The listing builds one solid part. Answer for the finished solid, in the listing's coordinates (mm). A direction names the side the tool comes from. Round coordinates to 2 decimals unless told otherwise and drop trailing zeros. Write each loop counter-clockwise with the first axis right and the second up, starting at its lowest first coordinate (ties: lowest second). Pieces come first, ordered by that corner, then holes. Notation, with made-up numbers: (39.5, 21) - (86.5, 21) arc R24 cw to (86.5, 43) - close; hole circle Ø7 at (-40, 82). An arc over 180 degrees is marked (long way). Return JSON: item names as keys, results as strings. Group by question number.
(1) Section D-D, the plane x = 7.75 is taken. Write down the section's boundary in (y, z), then the cut area to 3 significant figures.
(2) Section C-C, the plane z = 71 is taken. Write down the section's boundary in (x, y), then the cut area to 3 significant figures.
(3) Find the intervals of material crossed by line 1 along Z through (x, y) = (15, 1.4); line 2 along Y through (x, z) = (14.25, 40), in increasing order. Write a range as [from, to].
(4) Which of the six approach directions +Z, -Z, +X, -X, +Y, -Y give full straight-line access (tool end or side, diameter ignored) to faces 1 (the flat face through (16, 2.5, 93)), 2 (the cylindrical face through (1.27, 12.05, 17.7))?
(5) Determine the mould class of faces 3 (the cylindrical face through (15.867, 1.268, 171.895)), 4 (the cylindrical face through (18.996, 1.268, 12.676)), 5 (the flat face through (15, 0, 93)), 6 (the flat face through (2.5, 16, 93)) for opening direction X: +X half, -X half, draft (parallel to the pull), parting line (faces both ways), or undercut.
(6) Section B-B, the plane x = 15 is taken. Write down the section's boundary in (y, z), then the cut area to 3 significant figures.
(7) Each of these flat-tipped pins is pushed along its axis until it touches: pin 1 (13 mm diameter, centred on x = 15, z = 12.5, fed in from +Y); pin 2 (9 mm diameter, centred on y = 15, z = 15, fed in from +X); pin 3 (7 mm diameter, centred on x = 15, z = 175.8, fed in from -Y). Where does it stop, or does it pass through?
(8) Section A-A, the plane y = 15 is taken. Write down the section's boundary in (x, z).
```python
from build123d import *

# Parameters (mm, degrees)
BOSS_EXTRUDE1_DEPTH = 188.3
SKETCH2_R           = 4
CUT_EXTRUDE1_DEPTH  = 193.647709563
SKETCH3_R           = 4
CUT_EXTRUDE2_DEPTH  = 193.647709563


with BuildPart() as part:
    # Sketch1 → Boss-Extrude1 (new body)
    with BuildSketch(Plane.XY):
        Polygon((0, 0), (0, 30), (2.5, 30), (2.5, 2.5), (30, 2.5), (30, 0), align=None)
    extrude(amount=BOSS_EXTRUDE1_DEPTH)

    # Sketch2 → Cut-Extrude1 (cut, through all)
    with BuildSketch(Plane(origin=(0, 2.5, 0), x_dir=(1, 0, 0), z_dir=(0, 1, 0))):
        with Locations(Location((15, -12.5, 0), (0, 0, 180))):
            Circle(SKETCH2_R)
        with Locations(Location((15, -175.8, 0), (0, 0, 180))):
            Circle(SKETCH2_R)
    extrude(amount=-CUT_EXTRUDE1_DEPTH, mode=Mode.SUBTRACT)

    # Sketch3 → Cut-Extrude2 (cut, through all)
    with BuildSketch(Plane(origin=(2.5, 0, 0), x_dir=(0, 0, -1), z_dir=(1, 0, 0))):
        with Locations(Location((-15, 15, 0), (0, 0, 90))):
            Circle(SKETCH3_R)
        with Locations(Location((-173.3, 15, 0), (0, 0, 270))):
            Circle(SKETCH3_R)
    extrude(amount=-CUT_EXTRUDE2_DEPTH, mode=Mode.SUBTRACT)


solid = part.part
```
Working result:
{
 "1": {"outline": "(0, 0) - (2.5, 0) - (2.5, 188.3) - (0, 188.3) - close", "area": "471 mm^2"},
 "2": {"outline": "(0, 0) - (30, 0) - (30, 2.5) - (2.5, 2.5) - (2.5, 30) - (0, 30) - close", "area": "144 mm^2"},
 "3": {"line 1": "z = [0, 8.5], [16.5, 171.8], [179.8, 188.3]", "line 2": "y = [0, 2.5]"},
 "4": {"face 1": "+Z, -Z, +X, +Y", "face 2": "+X, -X"},
 "5": {"face 3": "undercut", "face 4": "undercut", "face 5": "draft", "face 6": "+X half"},
 "6": {"outline": "(0, 0) - (2.5, 0) - (2.5, 8.5) - (0, 8.5) - close; (0, 16.5) - (2.5, 16.5) - (2.5, 171.8) - (0, 171.8) - close; (0, 179.8) - (2.5, 179.8) - (2.5, 188.3) - (0, 188.3) - close", "area": "431 mm^2"},
 "7": {"pin 1": "stops at y = 2.5", "pin 2": "stops at x = 2.5", "pin 3": "passes through"},
 "8": {"outline": "(0, 0) - (2.5, 0) - (2.5, 11) - (0, 11) - close; (0, 19) - (2.5, 19) - (2.5, 169.3) - (0, 169.3) - close; (0, 177.3) - (2.5, 177.3) - (2.5, 188.3) - (0, 188.3) - close"}
}
